from build123d import *

# Parameters (mm, degrees)
SKETCH1_W               = 135
SKETCH1_H               = 135
BOSS_EXTRUDE1_DEPTH     = 3
BOSS_EXTRUDE2_DEPTH     = 10
SKETCH3_R               = 44.45
SKETCH3_R_2             = 41.45
BOSS_EXTRUDE3_DEPTH     = 15
CUT_EXTRUDE1_DEPTH      = 192.507180022
CUT_EXTRUDE1_DEPTH_BACK = 192.507180022
SKETCH4_R               = 1.1
CUT_EXTRUDE2_DEPTH      = 192.507180022
CUT_EXTRUDE2_DEPTH_BACK = 192.507180022
SKETCH5_R               = 3.5


with BuildPart() as part:
    # Sketch1 → Boss-Extrude1 (new body)
    with BuildSketch(Plane(origin=(0, 0, 0), x_dir=(1, 0, 0), z_dir=(0, 1, 0))):
        with Locations((67.5, 67.5)):
            Rectangle(SKETCH1_W, SKETCH1_H)
    extrude(amount=BOSS_EXTRUDE1_DEPTH)

    # Sketch2 → Boss-Extrude2 (add)
    with BuildSketch(Plane(origin=(0, 3, 0), x_dir=(1, 0, 0), z_dir=(0, 1, 0))):
        with BuildLine():
            ThreePointArc((50.907776173, 56.333169273), (52.06098052, 54.786358606), (53.357864376, 53.357864376))
            Line((53.357864376, 53.357864376), (81.642135624, 81.642135624))
            ThreePointArc((81.642135624, 81.642135624), (75.784522289, 85.703480174), (68.874647176, 87.452702703))
            ThreePointArc((68.874647176, 87.452702703), (67.5, 87.5), (66.125352824, 87.452702703))
            ThreePointArc((66.125352824, 87.452702703), (57.5, 84.820508076), (50.907776173, 78.666830727))
            ThreePointArc((50.907776173, 78.666830727), (50.179491924, 77.5), (49.533128997, 76.285871976))
            ThreePointArc((49.533128997, 76.285871976), (47.5, 67.5), (49.533128997, 58.714128024))
            ThreePointArc((49.533128997, 58.714128024), (50.179491924, 57.5), (50.907776173, 56.333169273))
        make_face()
        with BuildLine():
            Line((81.642135624, 81.642135624), (53.357864376, 53.357864376))
            ThreePointArc((53.357864376, 53.357864376), (59.215477711, 49.296519826), (66.125352824, 47.547297297))
            ThreePointArc((66.125352824, 47.547297297), (67.5, 47.5), (68.874647176, 47.547297297))
            ThreePointArc((68.874647176, 47.547297297), (77.5, 50.179491924), (84.092223827, 56.333169273))
            ThreePointArc((84.092223827, 56.333169273), (84.820508076, 57.5), (85.466871003, 58.714128024))
            ThreePointArc((85.466871003, 58.714128024), (86.985089428, 62.990976827), (87.5, 67.5))
            ThreePointArc((87.5, 67.5), (86.985089428, 72.009023173), (85.466871003, 76.285871976))
            ThreePointArc((85.466871003, 76.285871976), (84.820508076, 77.5), (84.092223827, 78.666830727))
            ThreePointArc((84.092223827, 78.666830727), (82.93901948, 80.213641394), (81.642135624, 81.642135624))
        make_face()
        with BuildLine():
            ThreePointArc((66.125352824, 87.452702703), (67.5, 87.5), (68.874647176, 87.452702703))
            ThreePointArc((68.874647176, 87.452702703), (67.5, 88), (66.125352824, 87.452702703))
        make_face()
        with BuildLine():
            ThreePointArc((68.874647176, 47.547297297), (67.5, 47), (66.125352824, 47.547297297))
            ThreePointArc((66.125352824, 47.547297297), (67.5, 47.5), (68.874647176, 47.547297297))
        make_face()
        with BuildLine():
            ThreePointArc((50.907776173, 56.333169273), (49.746479222, 57.25), (49.533128997, 58.714128024))
            ThreePointArc((49.533128997, 58.714128024), (50.179491924, 57.5), (50.907776173, 56.333169273))
        make_face()
        with BuildLine():
            ThreePointArc((85.466871003, 58.714128024), (85.253520778, 57.25), (84.092223827, 56.333169273))
            ThreePointArc((84.092223827, 56.333169273), (84.820508076, 57.5), (85.466871003, 58.714128024))
        make_face()
        with BuildLine():
            ThreePointArc((84.092223827, 78.666830727), (85.253520778, 77.75), (85.466871003, 76.285871976))
            ThreePointArc((85.466871003, 76.285871976), (84.820508076, 77.5), (84.092223827, 78.666830727))
        make_face()
        with BuildLine():
            ThreePointArc((49.533128997, 76.285871976), (49.746479222, 77.75), (50.907776173, 78.666830727))
            ThreePointArc((50.907776173, 78.666830727), (50.179491924, 77.5), (49.533128997, 76.285871976))
        make_face()
    extrude(amount=BOSS_EXTRUDE2_DEPTH)

    # Sketch3 → Boss-Extrude3 (add)
    with BuildSketch(Plane(origin=(0, 3, 0), x_dir=(1, 0, 0), z_dir=(0, 1, 0))):
        with Locations(Location((67.5, 67.5, 0), (0, 0, 90))):
            Circle(SKETCH3_R)
        with Locations(Location((67.5, 67.5, 0), (0, 0, 270))):
            Circle(SKETCH3_R_2, mode=Mode.SUBTRACT)
    extrude(amount=BOSS_EXTRUDE3_DEPTH)

    # Sketch4 → Cut-Extrude1 (cut, two sides: drawn at the far end of the back side and taken through both)
    with BuildSketch(Plane(origin=(0, 3, 0), x_dir=(1, 0, 0), z_dir=(0, 1, 0)).offset(-CUT_EXTRUDE1_DEPTH_BACK)):
        with Locations(Location((67.5, 97.5, 0), (0, 0, 270))):
            Circle(SKETCH4_R)
        with Locations(Location((97.5, 67.5, 0), (0, 0, 270))):
            Circle(SKETCH4_R)
        with Locations(Location((67.5, 37.5, 0), (0, 0, 270))):
            Circle(SKETCH4_R)
        with Locations(Location((37.5, 67.5, 0), (0, 0, 270))):
            Circle(SKETCH4_R)
    extrude(amount=CUT_EXTRUDE1_DEPTH + CUT_EXTRUDE1_DEPTH_BACK, mode=Mode.SUBTRACT)

    # Sketch5 → Cut-Extrude2 (cut, two sides: drawn at the far end of the back side and taken through both)
    with BuildSketch(Plane(origin=(0, 3, 0), x_dir=(1, 0, 0), z_dir=(0, 1, 0)).offset(-CUT_EXTRUDE2_DEPTH_BACK)):
        with Locations(Location((67.5, 120.5, 0), (0, 0, 270))):
            Circle(SKETCH5_R)
        with Locations(Location((104.976659403, 104.976659403, 0), (0, 0, 270))):
            Circle(SKETCH5_R)
        with Locations(Location((120.5, 67.5, 0), (0, 0, 270))):
            Circle(SKETCH5_R)
        with Locations(Location((104.976659403, 30.023340597, 0), (0, 0, 270))):
            Circle(SKETCH5_R)
        with Locations(Location((67.5, 14.5, 0), (0, 0, 270))):
            Circle(SKETCH5_R)
        with Locations(Location((30.023340597, 30.023340597, 0), (0, 0, 270))):
            Circle(SKETCH5_R)
        with Locations(Location((14.5, 67.5, 0), (0, 0, 270))):
            Circle(SKETCH5_R)
        with Locations(Location((30.023340597, 104.976659403, 0), (0, 0, 270))):
            Circle(SKETCH5_R)
    extrude(amount=CUT_EXTRUDE2_DEPTH + CUT_EXTRUDE2_DEPTH_BACK, mode=Mode.SUBTRACT)


solid = part.part
Source: CAD feature listing. Evaluate the final solid. Frame: model axes, mm. A direction names the side the tool comes from. Give positions to 0.01 mm unless a question says otherwise; leave off trailing zeros. Write each loop counter-clockwise with the first axis right and the second up, starting at its lowest first coordinate (ties: lowest second). Pieces come first, ordered by that corner, then holes. Notation, with made-up numbers: M -16,-32 L 6,-32 A20 ccw 6,-19 Z; hole C 18,70.25 d8. An arc over 180 degrees is marked long. Answer as a JSON object with one key per item and string values.
Q1. Mould query, pull axis X, two halves, no side actions, for faces 3 (the face through (54, 18, -107)), 4 (the face through (77.39, 7.93, -50.116)), 5 (the face through (0, 1, -67)), 6 (the face through (54.148, 10.395, -109.897)). Classes: +X half, -X half, draft (parallel to the pull), parting line (faces both ways), or undercut.
Geometry check:
{"face 3": "draft", "face 4": "undercut", "face 5": "-X half", "face 6": "parting line"}
Q2. Cut plane D-D, the plane z = -92.5. Return the cut outline in (x, y).
Geometry check:
{"outline": "M 0,0 L 135,0 L 135,3 L 104.25,3 L 104.25,18 L 100.56,18 L 100.56,3 L 34.44,3 L 34.44,18 L 30.75,18 L 30.75,3 L 0,3 Z"}
Q3. Cut plane C-C, the plane x = 73. Return the cut outline in (y, z), then the cut area to 3 significant figures.
Geometry check:
{"outline": "M 0,-135 L 3,-135 L 3,-111.61 L 18,-111.61 L 18,-108.58 L 3,-108.58 L 3,-86.73 L 13,-86.73 L 13,-48.27 L 3,-48.27 L 3,-26.42 L 18,-26.42 L 18,-23.39 L 3,-23.39 L 3,0 L 0,0 Z", "area": "880 mm^2"}
Q4. Access query for faces 1 (the face through (79.95, 10.395, -27.964)), 2 (the face through (107.34, 1.48, -107.56)). Directions: +Z, -Z, +X, -X, +Y, -Y. A direction counts if a zero-diameter tool reaches every point of the face in a straight line with its end or side. Return the directions, or none.
Geometry check:
{"face 1": "+Y", "face 2": "+Y, -Y"}
Q5. Cut plane A-A, the plane y = 10. Return the cut outline in (x, z), then the cut area to 3 significant figures.
Geometry check:
{"outline": "C 67.5,-67.5 d88.9; M 49.53,-76.29 A2 ccw 50.91,-78.67 A20 ccw 66.13,-87.45 A2 ccw 68.87,-87.45 A20 ccw 84.09,-78.67 A2 ccw 85.47,-76.29 A20 ccw 85.47,-58.71 A2 ccw 84.09,-56.33 A20 ccw 68.87,-47.55 A2 ccw 66.13,-47.55 A20 ccw 50.91,-56.33 A2 ccw 49.53,-58.71 A20 ccw Z; hole C 67.5,-67.5 d82.9", "area": "2,070 mm^2"}
Q6. Cut plane B-B, the plane z = -120.5. Return the cut outline in (x, y), then the cut area to 3 significant figures.
Geometry check:
{"outline": "M 0,0 L 64,0 L 64,3 L 0,3 Z; M 71,0 L 135,0 L 135,3 L 71,3 Z", "area": "384 mm^2"}
Q7. Ray query, line 1 along Z through (x, y) = (67.5, 1.9); line 2 along X through (y, z) = (10.5, -67.5); line 3 along X through (y, z) = (1, -67.5). Return the intervals inside material, ascending.
Geometry check:
{"line 1": "z = -135 to -124, -117 to -98.6, -96.4 to -38.6, -36.4 to -18, -11 to 0", "line 2": "x = 23.05 to 26.05, 47.5 to 87.5, 108.95 to 111.95", "line 3": "x = 0 to 11, 18 to 36.4, 38.6 to 96.4, 98.6 to 117, 124 to 135"}
Q8. Contact query for flat-ended pins moving along their axis: P1, Ø11, axis at x = 67.5, z = -120.5, coming from the +Y side; P2, Ø25, axis at x = 70, z = -54.5, coming from the +Y side; P3, Ø1.8, axis at x = 67.5, z = -97.5, coming from the +Y side; P4, Ø4, axis at y = 7.5, z = -31, coming from the -X side. Output: stop coordinate, or through.
Geometry check:
{"P1": "stops at y = 3", "P2": "stops at y = 13", "P3": "passes through", "P4": "stops at x = 39.47"}
